Study the drawing (mm; zero at the part's minimum x, y, z) and answer. A direction names the side the tool comes from. Coordinates: 2 decimals unless noted, no trailing zeros. Order: outer loops, then holes, each group sorted by start corner. A loop starts at its lowest first (then second) coordinate and runs counter-clockwise, first axis right, second up.
1. The part is cut by section A-A, the plane x = 2.5. Give the vertices of the cut face in (y, z).
2. A tool of negligible diameter and unlimited length cuts with its end or side. For the marked faces 1, 2 and 3, from which of +Z, -Z, +X, -X, +Y, -Y can it reach the whole face along a straight path? Write none if from no direction.
3. Flat-ended cylindrical pins translate along their axes: pin 1 Ø1.5 at (x, z) = (3.5, 6) entering from -Y; pin 2 Ø4 at (x, z) = (4.5, 2) entering from -Y; pin 3 Ø6 at (x, z) = (12.5, 3) entering from +Y; pin 4 Ø2 at (y, z) = (6, 3) entering from -X. Find the tip coordinate at first contact, or state that the pin passes through.
4. Find the intervals of material crossed by probe 1 along Y at (x, z) = (7.5, 4.5); probe 2 along X at (y, z) = (12, 7); probe 3 along Y at (x, z) = (2, 5.25), in increasing order.
5. The part is cut by section D-D, the plane y = 5.5. Give the vertices of the cut face in (x, z), then the cut area to 3 significant figures.
6. The part is cut by section C-C, the plane x = 15. Give the vertices of the cut face in (y, z), then the cut area to 3 significant figures.
7. The part is cut by section B-B, the plane z = 11.5. Give the vertices of the cut face in (x, y).
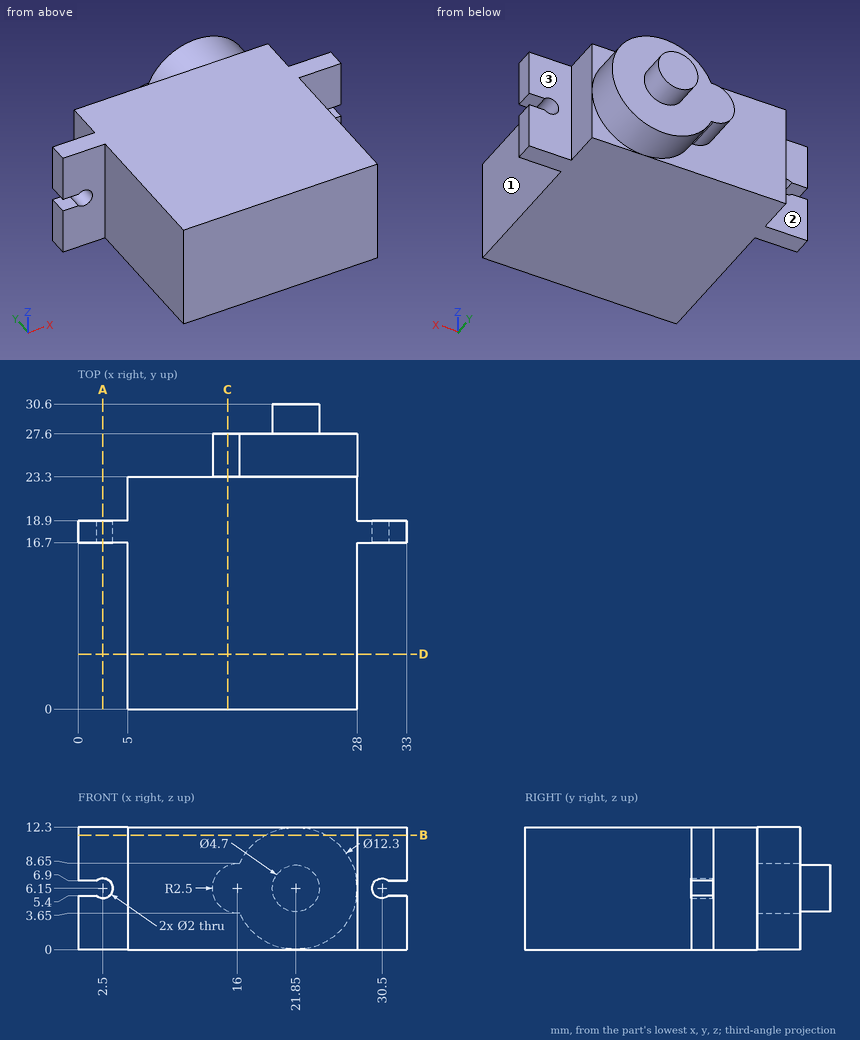
Geometry says:
1. outline: (16.7, 0) - (18.9, 0) - (18.9, 5.15) - (16.7, 5.15) - close; (16.7, 7.15) - (18.9, 7.15) - (18.9, 12.3) - (16.7, 12.3) - close
2. face 1: +Z, -Z, +X, -Y
2. face 2: +Z, -Z, -X, +Y
2. face 3: +Z, -Z, +X, +Y
3. pin 1: stops at y = 16.7
3. pin 2: stops at y = 0
3. pin 3: stops at y = 27.6
3. pin 4: stops at x = 5
4. probe 1: y = 0 to 23.3
4. probe 2: x = 5 to 28
4. probe 3: y = 16.7 to 18.9
5. outline: (5, 0) - (28, 0) - (28, 12.3) - (5, 12.3) - close
5. area: 283 mm2
6. outline: (0, 0) - (23.3, 0) - (23.3, 3.86) - (27.6, 3.86) - (27.6, 8.44) - (23.3, 8.44) - (23.3, 12.3) - (0, 12.3) - close
6. area: 306 mm2
7. outline: (0, 16.7) - (5, 16.7) - (5, 0) - (28, 0) - (28, 16.7) - (33, 16.7) - (33, 18.9) - (28, 18.9) - (28, 23.3) - (24.88, 23.3) - (24.88, 27.6) - (18.82, 27.6) - (18.82, 23.3) - (5, 23.3) - (5, 18.9) - (0, 18.9) - close
